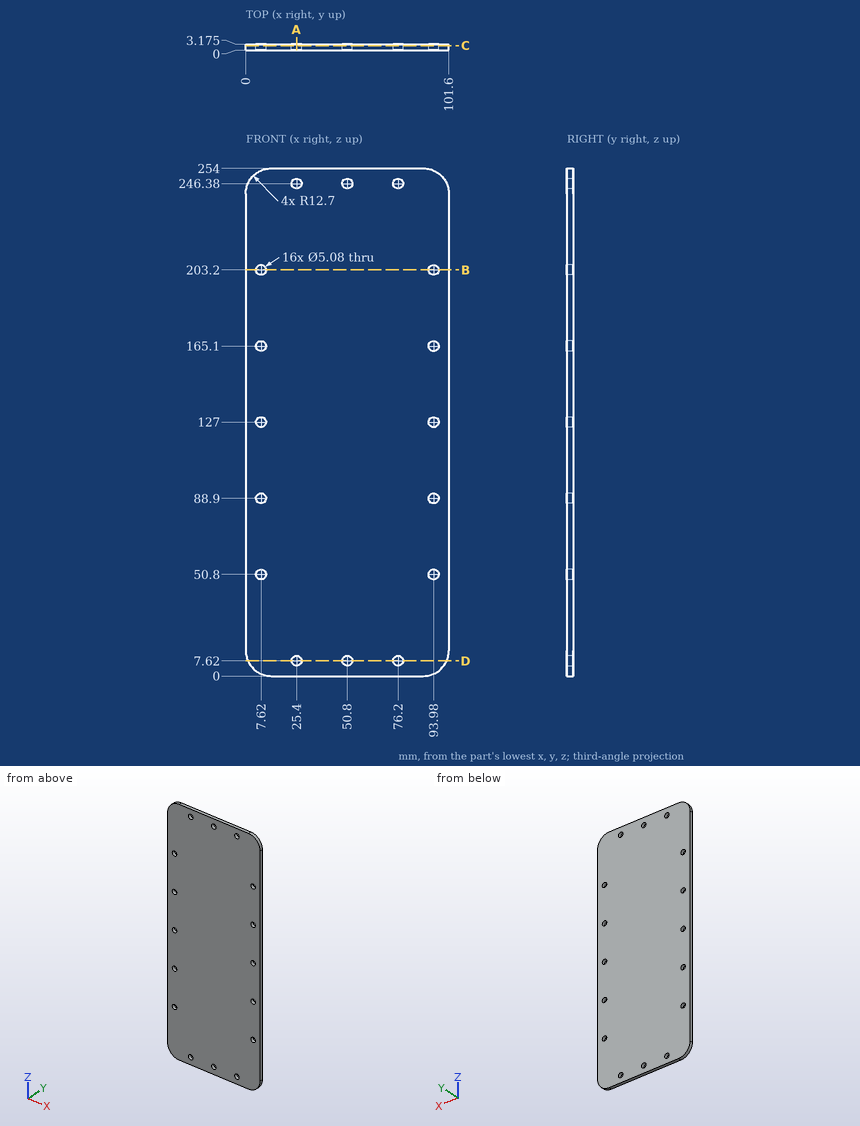
Job drawing, mm, ordinate dimensions from the low corner. One solid piece. Give positions to 0.01 mm unless a question says otherwise; leave off trailing zeros. Order: outer loops, then holes, each group sorted by start corner. A loop starts at its lowest first (then second) coordinate and runs counter-clockwise, first axis right, second up. Notation, with made-up numbers: M 81.5,81.5 L 98.5,81.5 A19 cw 98.5,90.5 Z; hole C 56.25,41 d3. An arc over 180 degrees is marked long. Return JSON: item names as keys, results as strings.
Q1. Band-saw the part on D-D (z = 7.62). Give the cut face in (x, y) (3 decimals), then the cut area to 3 significant figures.
Answer list:
{"outline": "M 1.06,0 L 22.86,0 L 22.86,3.175 L 1.06,3.175 Z; M 27.94,0 L 48.26,0 L 48.26,3.175 L 27.94,3.175 Z; M 53.34,0 L 73.66,0 L 73.66,3.175 L 53.34,3.175 Z; M 78.74,0 L 100.54,0 L 100.54,3.175 L 78.74,3.175 Z", "area": "267 mm^2"}
Q2. Band-saw the part on B-B (z = 203.2). Give the cut face in (x, y) (3 decimals).
Answer list:
{"outline": "M 0,0 L 5.08,0 L 5.08,3.175 L 0,3.175 Z; M 10.16,0 L 91.44,0 L 91.44,3.175 L 10.16,3.175 Z; M 96.52,0 L 101.6,0 L 101.6,3.175 L 96.52,3.175 Z"}
Q3. Band-saw the part on A-A (x = 25.4). Give the cut face in (y, z) (3 decimals).
Answer list:
{"outline": "M 0,0 L 3.175,0 L 3.175,5.08 L 0,5.08 Z; M 0,10.16 L 3.175,10.16 L 3.175,243.84 L 0,243.84 Z; M 0,248.92 L 3.175,248.92 L 3.175,254 L 0,254 Z"}
Q4. Wall check: probe 1 along X at (y, z) = (0.95, 127); probe 2 along X at (y, z) = (2.05, 246.38); probe 3 along X at (y, z) = (1, 90.5). Give the ranges that are in metal, low to high. Write a range as from..to.
Answer list:
{"probe 1": "x = 0..5.08, 10.16..91.44, 96.52..101.6", "probe 2": "x = 1.06..22.86, 27.94..48.26, 53.34..73.66, 78.74..100.54", "probe 3": "x = 0..5.65, 9.59..92.01, 95.95..101.6"}
Q5. Band-saw the part on C-C (y = 2.3). Count the separate pieces of the cut face and the enclosed holes in it, then the cut area to 3 significant figures.
Answer list:
{"separate pieces": "1", "enclosed holes": "16", "area": "25,300 mm^2"}
